Check sheet for the modelled part. Datum: model origin and axes. Units: mm. A direction names the side the tool comes from. Round coordinates to 2 decimals unless told otherwise and drop trailing zeros. Order: outer loops, then holes, each group sorted by start corner. A loop starts at its lowest first (then second) coordinate and runs counter-clockwise, first axis right, second up. Notation, with made-up numbers: (18.25, 38) -> (68.25, 38) arc R22 cw to (68.25, 53) -> close; hole circle Ø6 at (19, -37.5). An arc over 180 degrees is marked (long way). Use CSV: the item, a comma, the result in double quotes.
```python
from build123d import *

# Parameters (mm, degrees)
EXTRUDE_1_DEPTH          = 4.4
CUT_EXTRUDE_1_DEPTH      = 0.6
FILLET_1_R               = 1.5
SKETCH_3_W               = 5
SKETCH_3_H               = 9
EXTRUDE_2_DEPTH          = 14.5
FILLET_2_R               = 4.5
CUT_EXTRUDE_2_DEPTH      = 57.417976641
CUT_EXTRUDE_2_DEPTH_BACK = 57.417976641
SKETCH_4_R               = 1.55
CUT_EXTRUDE_3_DEPTH      = 55.68383811
CUT_EXTRUDE_3_DEPTH_BACK = 55.68383811
SKETCH_5_R               = 1.25


with BuildPart() as part:
    # 스케치1 → 보스-돌출1 (new body)
    with BuildSketch(Plane(origin=(0, 0, 0), x_dir=(1, 0, 0), z_dir=(0, 1, 0))):
        Polygon((27.293187568, -27.293187568), (37.283187568, -9.99), (37.283187568, 9.99), (27.293187568, 27.293187568), (9.99, 37.283187568), (-9.99, 37.283187568), (-27.293187568, 27.293187568), (-37.283187568, 9.99), (-37.283187568, -9.99), (-27.293187568, -27.293187568), (-9.99, -37.283187568), (9.99, -37.283187568), align=None)
    extrude(amount=EXTRUDE_1_DEPTH)

    # 스케치2 → 컷-돌출1 (cut)
    with BuildSketch(Plane(origin=(0, 4.4, 0), x_dir=(1, 0, 0), z_dir=(0, 1, 0))):
        Polygon((-26.120860153, 26.120860153), (-35.681758538, 9.560898385), (-35.681758538, -9.560898385), (-26.120860153, -26.120860153), (-9.560898385, -35.681758538), (9.560898385, -35.681758538), (26.120860153, -26.120860153), (35.681758538, -9.560898385), (35.681758538, 9.560898385), (26.120860153, 26.120860153), (9.560898385, 35.681758538), (-9.560898385, 35.681758538), align=None)
        Polygon((24.656758538, -24.656758538), (33.681758538, -9.025), (33.681758538, 9.025), (24.656758538, 24.656758538), (9.025, 33.681758538), (-9.025, 33.681758538), (-24.656758538, 24.656758538), (-33.681758538, 9.025), (-33.681758538, -9.025), (-24.656758538, -24.656758538), (-9.025, -33.681758538), (9.025, -33.681758538), align=None, mode=Mode.SUBTRACT)
    extrude(amount=-CUT_EXTRUDE_1_DEPTH, mode=Mode.SUBTRACT)

    # 필렛1
    fillet_1_edges = [part.edges().sort_by_distance(p)[0] for p in [
        (0, 0, 37.283187568),
        (-18.641593784, 0, 32.288187568),
        (37.283187568, 4.4, 0),
        (-32.288187568, 0, 18.641593784),
        (-37.283187568, 0, 0),
        (-32.288187568, 0, -18.641593784),
        (-18.641593784, 0, -32.288187568),
        (0, 0, -37.283187568),
        (18.641593784, 0, -32.288187568),
        (32.288187568, 0, -18.641593784),
        (37.283187568, 0, 0),
        (32.288187568, 0, 18.641593784),
        (18.641593784, 0, 32.288187568),
        (32.288187568, 4.4, -18.641593784),
        (18.641593784, 4.4, -32.288187568),
        (0, 4.4, -37.283187568),
        (-18.641593784, 4.4, -32.288187568),
        (-32.288187568, 4.4, -18.641593784),
        (-37.283187568, 4.4, 0),
        (-32.288187568, 4.4, 18.641593784),
        (-18.641593784, 4.4, 32.288187568),
        (0, 4.4, 37.283187568),
        (18.641593784, 4.4, 32.288187568),
        (32.288187568, 4.4, 18.641593784),
    ]]
    fillet(fillet_1_edges, radius=FILLET_1_R)

    # 스케치3 → 보스-돌출2 (add)
    with BuildSketch(Plane.XZ):
        with Locations((0, -15)):
            Rectangle(SKETCH_3_W, SKETCH_3_H)
        with Locations((0, 15)):
            Rectangle(SKETCH_3_W, SKETCH_3_H)
    extrude(amount=EXTRUDE_2_DEPTH)

    # 필렛2
    fillet_2_edges = [part.edges().sort_by_distance(p)[0] for p in [
        (0, -14.5, -19.5),
        (0, -14.5, -10.5),
        (0, -14.5, 19.5),
        (0, -14.5, 10.5),
    ]]
    fillet(fillet_2_edges, radius=FILLET_2_R - 0.0001)  # a hair under: the kernel refuses the full size

    # 스케치4 → 컷-돌출2 (cut, two sides: drawn at the far end of the back side and taken through both)
    with BuildSketch(Plane.ZY.offset(2.5).offset(-CUT_EXTRUDE_2_DEPTH_BACK)):
        with Locations((-15, -10)):
            Circle(SKETCH_4_R)
        with Locations((15, -10)):
            Circle(SKETCH_4_R)
    extrude(amount=CUT_EXTRUDE_2_DEPTH + CUT_EXTRUDE_2_DEPTH_BACK, mode=Mode.SUBTRACT)

    # 스케치5 → 컷-돌출3 (cut, two sides: drawn at the far end of the back side and taken through both)
    with BuildSketch(Plane.XZ.offset(-CUT_EXTRUDE_3_DEPTH_BACK)):
        with Locations(Location((17.7, 0, 0), (0, 0, 270))):
            Circle(SKETCH_5_R)
    extrude(amount=CUT_EXTRUDE_3_DEPTH + CUT_EXTRUDE_3_DEPTH_BACK, mode=Mode.SUBTRACT)


solid = part.part
```
Q1. Go/stop test with flat-tipped pins: pin 1 (1.5 mm diameter, centred on y = 2, z = -16, fed in from +X); pin 2 (1.5 mm diameter, centred on x = 0, y = -3.5, fed in from +Z); pin 3 (0.5 mm diameter, centred on x = 3, y = 4, fed in from +Z). Record where each tip stops, or that it passes through.
Result sheet:
pin 1,"stops at x = 34.25"
pin 2,"stops at z = 19.5"
pin 3,"stops at z = 37.02"
Q2. Access from +Z, -Z, +X, -X, +Y, -Y to the whole of each face (thin tool, end or side, straight path). Record for faces 4 (the face through (0, -5, -19.5)), 5 (the face through (0, -5, 19.5)), 6 (the face through (-29.106, 4.104, -16.95)).
Result sheet:
face 4,"-Z, +X, -X, -Y"
face 5,"+Z, +X, -X, -Y"
face 6,"+Y"
Q3. Mould release check, pull along Z, two halves, no side actions. Record for faces 1 (the face through (-16.731, 4.104, -29.232)), 2 (the face through (-18.76, 2.19, 32.22)), 3 (the face through (-18.54, 0.43, -31.83)): pulls with the +Z half, pulls with the -Z half, needs draft (parallel to the pull), parting line crosses it, or undercut.
Result sheet:
face 1,"undercut"
face 2,"pulls with the +Z half"
face 3,"pulls with the -Z half"
Q4. Scan lines: L1, parallel to Z at x = 0.3, y = -10; L2, parallel to Y at x = 0, z = 15; L3, parallel to Y at x = -6.5, z = -18. Record each from-to range of solid material in increasing order.
Result sheet:
L1,"z = -19.5 to -16.55, -13.45 to -10.5, 10.5 to 13.45, 16.55 to 19.5"
L2,"y = -14.5 to -11.55, -8.45 to 4.4"
L3,"y = 0 to 4.4"
Q5. Sectioned sample at C-C, the plane z = -6.5. Enter the section's corners in (x, y), then the cut area to 3 significant figures.
Result sheet:
outline,"(-37.28, 1.5) arc R1.5 ccw to (-35.78, 0) -> (35.78, 0) arc R1.5 ccw to (37.28, 1.5) -> (37.28, 2.9) arc R1.5 ccw to (35.78, 4.4) -> (35.68, 4.4) -> (35.68, 3.8) -> (33.68, 3.8) -> (33.68, 4.4) -> (-33.68, 4.4) -> (-33.68, 3.8) -> (-35.68, 3.8) -> (-35.68, 4.4) -> (-35.78, 4.4) arc R1.5 ccw to (-37.28, 2.9) -> close"
area,"324 mm^2"
Q6. Sectioned sample at A-A, the plane y = -7.5. Enter the section's corners in (x, z).
Result sheet:
outline,"(-2.5, -19.5) -> (2.5, -19.5) -> (2.5, -10.5) -> (-2.5, -10.5) -> close; (-2.5, 10.5) -> (2.5, 10.5) -> (2.5, 19.5) -> (-2.5, 19.5) -> close"
Q7. Sectioned sample at B-B, the plane x = 0. State how many separate pieces and enclosed holes the cut face has, then the cut area to 3 significant figures.
Result sheet:
separate pieces,"1"
enclosed holes,"2"
area,"552 mm^2"
